```python
from build123d import *

# Parameters (mm, degrees)
HEX_2_DEPTH = 1.1176


with BuildPart() as part:
    # BodySke → BaseBody (revolve)
    with BuildSketch(Plane.XY):
        with BuildLine():
            Line((14.5542, 0), (14.5542, 1.28016))
            Line((14.5542, 1.28016), (14.08176, 1.7526))
            Line((14.08176, 1.7526), (1.8542, 1.7526))
            Line((1.8542, 1.7526), (1.8542, 3.3274))
            Line((1.8542, 3.3274), (1.4732, 3.3274))
            ThreePointArc((1.4732, 3.3274), (0.616396771, 2.601989501), (0, 1.6637))
            Line((0, 1.6637), (0, 0))
            Line((0, 0), (14.5542, 0))
        make_face()
    revolve(axis=Axis((0, 0, 0), (1, 0, 0)))

    # Sketch2 → PreBroach (revolve, cut)
    with BuildSketch(Plane.XY):
        Polygon((0, 0.9906), (1.1176, 0.9906), (1.689523177, 0), (0, 0), align=None)
    revolve(axis=Axis((0, 0, 0), (1, 0, 0)), mode=Mode.SUBTRACT)

    # Sketch3 → Hex 2 (cut)
    with BuildSketch(Plane(origin=(0, 0, 0), x_dir=(0, 0, -1), z_dir=(1, 0, 0))):
        Polygon((-0.9906, -0.571923177), (-0.9906, 0.571923177), (0, 1.143846353), (0.9906, 0.571923177), (0.9906, -0.571923177), (0, -1.143846353), align=None)
    extrude(amount=HEX_2_DEPTH, mode=Mode.SUBTRACT)


solid = part.part
```
The model under review builds one solid part; all positions refer to its coordinate system, in mm. A direction names the side the tool comes from. Coordinates: 2 decimals unless noted, no trailing zeros. Order: outer loops, then holes, each group sorted by start corner. A loop starts at its lowest first (then second) coordinate and runs counter-clockwise, first axis right, second up. Notation, with made-up numbers: (12.5, 68.25) -> (32.5, 68.25) arc R26 cw to (32.5, 91.25) -> close; hole circle Ø5 at (-19.75, 72). An arc over 180 degrees is marked (long way). Answer in a Markdown table with one row per item. Add a question column.
Item 1: Clearance check with flat-ended pins moving along their axes: pin 1 (0.6 mm diameter, centred on x = 0.5, y = 0, fed in from -Z); pin 2 (1.2 mm diameter, centred on x = 0.5, y = 0, fed in from +Z); pin 3 (3 mm diameter, centred on x = 3, y = -2.5, fed in from +Z). State where each tip first meets the part, or that it passes through.
Item 2: Machinability: for faces 1 (the flat face through (1.854, -1.4, -1.4)), 2 (the cylindrical face through (1.66, -0.72, -3.25)), 3 (the flat face through (0.6, 0, 0.991)), which of the approach directions +Z, -Z, +X, -X, +Y, -Y give a long, thin tool a straight path to every point of the face, cutting with its end or side? Answer none if there is none.
Item 3: We need section B-B on z = 2.5. Write out the cut boundary in (x, y), plus the area to 3 significant figures.
Item 4: We need section C-C on y = 2.75. Write out the cut boundary in (x, z), plus the area to 3 significant figures.
Item 5: To check wall thickness, follow probe 1 along Z at (x, y) = (9.25, 0); probe 2 along Z at (x, y) = (13.75, 0.5); probe 3 along X at (y, z) = (-2.25, 1.75). State the ranges of each line that lie inside material, in increasing order.
Item 6: We need section A-A on x = 9.5. Write out the cut boundary in (y, z).
Item 7: Mouldability with a two-part tool opening along Z and no side actions: class faces 4 (the flat face through (0.55, -0.86, 0.49)), 5 (the flat face through (0.55, 0.86, -0.49)), 6 (the cylindrical face through (7.88, 1.67, 0.53)), 7 (the flat face through (14.554, 0, 0)) as +Z half, -Z half, draft (parallel to the pull), parting line (faces both ways), or undercut.
Final values:
| question | item | result |
|---|---|---|
| 1 | pin 1 | stops at z = -2.8 |
| 1 | pin 2 | stops at z = 3.06 |
| 1 | pin 3 | stops at z = 2.95 |
| 2 | face 1 | +X |
| 2 | face 2 | +X, -X |
| 2 | face 3 | -X |
| 3 | outline | (1.47, -2.2) -> (1.85, -2.2) -> (1.85, 2.2) -> (1.47, 2.2) arc R3.03 ccw to start |
| 3 | area | 4.54 mm2 |
| 4 | outline | (1.47, -1.87) -> (1.85, -1.87) -> (1.85, 1.87) -> (1.47, 1.87) arc R2.8 ccw to start |
| 4 | area | 3.27 mm2 |
| 5 | probe 1 | z = -1.75 to 1.75 |
| 5 | probe 2 | z = -1.68 to 1.68 |
| 5 | probe 3 | x = 0.86 to 1.85 |
| 6 | outline | circle Ø3.51 at (0, 0) |
| 7 | face 4 | undercut |
| 7 | face 5 | undercut |
| 7 | face 6 | parting line |
| 7 | face 7 | draft |
